Geometry check sheet. Reference: the model listing, model coordinates, mm. A direction names the side the tool comes from. Coordinates: 2 decimals unless noted, no trailing zeros. Loops run counter-clockwise (first coordinate to the right, second up) from the corner with the lowest first, then second, coordinate; pieces in that order, holes last.
from build123d import *

# Parameters (mm, degrees)
EXTRU_MINCE1_DEPTH      = 35
ESQUISSE2_R             = 1.75
ENL_V_MAT_EXTRU_1_DEPTH = 10
CONG_1_R                = 2
ESQUISSE3_R             = 1.5
ENL_V_MAT_EXTRU_2_DEPTH = 10
ESQUISSE4_R             = 1.5
ENL_V_MAT_EXTRU_3_DEPTH = 10


with BuildPart() as part:
    # Esquisse1 → Extru.-Mince1 (new body)
    with BuildSketch(Plane.XY):
        Polygon((0, 120), (0, 0), (150, 0), (150, -3), (-3, -3), (-3, 120), align=None)
    extrude(amount=EXTRU_MINCE1_DEPTH)

    # Esquisse2 → Enlèv. mat.-Extru.1 (cut)
    with BuildSketch(Plane(origin=(0, 0, 0), x_dir=(1, 0, 0), z_dir=(0, 1, 0))):
        with Locations(Location((124, -17.5, 0), (0, 0, 270))):
            Circle(ESQUISSE2_R)
        with Locations(Location((136, -17.5, 0), (0, 0, 270))):
            Circle(ESQUISSE2_R)
    extrude(amount=-ENL_V_MAT_EXTRU_1_DEPTH, mode=Mode.SUBTRACT)

    # Congé1
    cong_1_edges = [part.edges().sort_by_distance(p)[0] for p in [
        (-1.5, 120, 35),
        (-1.5, 120, 0),
        (150, -1.5, 0),
        (150, -1.5, 35),
        (-3, -3, 17.5),
    ]]
    fillet(cong_1_edges, radius=CONG_1_R)

    # Esquisse3 → Enlèv. mat.-Extru.2 (cut)
    with BuildSketch(Plane(origin=(0, 0, 0), x_dir=(1, 0, 0), z_dir=(0, 1, 0))):
        with Locations(Location((36.8, -17.5, 0), (0, 0, 270))):
            Circle(ESQUISSE3_R)
        with Locations(Location((57.8, -17.5, 0), (0, 0, 270))):
            Circle(ESQUISSE3_R)
    extrude(amount=-ENL_V_MAT_EXTRU_2_DEPTH, mode=Mode.SUBTRACT)

    # Esquisse4 → Enlèv. mat.-Extru.3 (cut)
    with BuildSketch(Plane(origin=(0, 0, 0), x_dir=(0, 0, -1), z_dir=(1, 0, 0))):
        with Locations((-17.5, 36.8)):
            Circle(ESQUISSE4_R)
        with Locations((-17.5, 57.8)):
            Circle(ESQUISSE4_R)
    extrude(amount=-ENL_V_MAT_EXTRU_3_DEPTH, mode=Mode.SUBTRACT)


solid = part.part
1) Section check A-A on x = 136. Record the cut outline in (y, z), and give its area (3 significant figures).
Data:
outline: (-3, 0) - (0, 0) - (0, 15.75) - (-3, 15.75) - close; (-3, 19.25) - (0, 19.25) - (0, 35) - (-3, 35) - close
area: 94.5 mm2
2) Access from +Z, -Z, +X, -X, +Y, -Y to the whole of each face (thin tool, end or side, straight path). Record for faces 4 (the flat face through (74, 0, 17)), 5 (the flat face through (76, -3, 17)).
Data:
face 4: +Z, -Z, +X, +Y
face 5: +Z, -Z, +X, -X, -Y
3) Section check C-C on y = 112. Record the cut outline in (x, z).
Data:
outline: (-3, 0) - (0, 0) - (0, 35) - (-3, 35) - close
4) Mould release check, pull along Z, two halves, no side actions. Record for faces 1 (the flat face through (0, 61, 17)), 2 (the flat face through (72.9, -0.5, 0)), 3 (the cylindrical face through (36.87, -1.48, 16)): +Z half, -Z half, draft (parallel to the pull), parting line (faces both ways), or undercut.
Data:
face 1: draft
face 2: -Z half
face 3: undercut
5) Section check B-B on z = 5.5. Record the cut outline in (x, y).
Data:
outline: (-3, -1) arc R2 ccw to (-1, -3) - (150, -3) - (150, 0) - (0, 0) - (0, 120) - (-3, 120) - close
6) Material ranges on probe 1 along Y at (x, z) = (-0.75, 17.5); probe 2 along X at (y, z) = (-1.4, 17.5); probe 3 along Z at (x, y) = (124, -2.05), recorded low to high.
Data:
probe 1: y = -3 to 35.3, 38.3 to 56.3, 59.3 to 120
probe 2: x = -2.96 to 35.3, 38.3 to 56.3, 59.3 to 122.25, 125.75 to 134.25, 137.75 to 150
probe 3: z = 0 to 15.75, 19.25 to 35
7) Depth check by flat-ended pin: pin 1 (1.5 mm diameter, centred on x = 78.5, z = 13.5, fed in from +Y); pin 2 (17.5 mm diameter, centred on y = 39, z = 16, fed in from +X); pin 3 (2 mm diameter, centred on x = 124, z = 17.5, fed in from -Y). Enter the tip coordinate at first touch or a pass-through.
Data:
pin 1: stops at y = 0
pin 2: stops at x = 0
pin 3: passes through
